from build123d import *

# Parameters (mm, degrees)
SKETCH1_R           = 4
BOSS_EXTRUDE1_DEPTH = 4


with BuildPart() as part:
    # Sketch1 → Boss-Extrude1 (new body)
    with BuildSketch(Plane.XY):
        Polygon((-20, 25), (20, 25), (20, 29), (40, 29), (40, 25), (40, -25), (40, -29), (20, -29), (20, -25), (-20, -25), (-20, -29), (-40, -29), (-40, -25), (-40, 25), (-40, 29), (-20, 29), align=None)
        with Locations((30, 15.5)):
            Circle(SKETCH1_R, mode=Mode.SUBTRACT)
        with Locations(Location((-30, 15.5, 0), (0, 0, 180))):
            Circle(SKETCH1_R, mode=Mode.SUBTRACT)
        with Locations((-30, -15.5)):
            Circle(SKETCH1_R, mode=Mode.SUBTRACT)
        with Locations(Location((30, -15.5, 0), (0, 0, 180))):
            Circle(SKETCH1_R, mode=Mode.SUBTRACT)
    extrude(amount=BOSS_EXTRUDE1_DEPTH)


solid = part.part
Work out the finished part from the listing and answer in its coordinate system (mm). A direction names the side the tool comes from. Round coordinates to 2 decimals unless told otherwise and drop trailing zeros. Order: outer loops, then holes, each group sorted by start corner. A loop starts at its lowest first (then second) coordinate and runs counter-clockwise, first axis right, second up. Notation, with made-up numbers: M -1,-24 L 28,-24 A13 cw 28,-12 Z; hole C 68.25,-5 d4. An arc over 180 degrees is marked long. One line per item, written item: value.
Q1. Determine the mould class of faces 4 (the face through (-40, 0, 2)), 5 (the face through (30, 29, 2)), 6 (the face through (27.05, 18.2, 1.97)) for opening direction X: released by +X, released by -X, zero draft, split by the parting line, or undercut.
Derived:
face 4: released by -X
face 5: zero draft
face 6: undercut
Q2. Straight lines are drawn through the part: line 1 (Y direction, x = 30, z = 2.1); line 2 (X direction, y = 26, z = 0.4); line 3 (Y direction, x = 31, z = 1.55). For each, find the intervals that lie inside material, in ascending order.
Derived:
line 1: -29 to -19.5, -11.5 to 11.5, 19.5 to 29
line 2: -40 to -20, 20 to 40
line 3: -29 to -19.37, -11.63 to 11.63, 19.37 to 29
Q3. Find section C-C on z = 2.9. Write down the section's boundary in (x, y), then the cut area to 3 significant figures.
Derived:
outline: M -40,-29 L -20,-29 L -20,-25 L 20,-25 L 20,-29 L 40,-29 L 40,29 L 20,29 L 20,25 L -20,25 L -20,29 L -40,29 Z; hole C -30,-15.5 d8; hole C -30,15.5 d8; hole C 30,-15.5 d8; hole C 30,15.5 d8
area: 4,120 mm²
Q4. Find section B-B on y = -15.5. Write down the section's boundary in (x, z).
Derived:
outline: M -40,0 L -34,0 L -34,4 L -40,4 Z; M -26,0 L 26,0 L 26,4 L -26,4 Z; M 34,0 L 40,0 L 40,4 L 34,4 Z
Q5. Flat-ended cylindrical pins translate along their axes: pin 1 (2 mm diameter, centred on x = -6.5, z = 3, fed in from +Y); pin 2 (7 mm diameter, centred on x = 30, y = -15.5, fed in from -Z) (3 decimals). Find the tip coordinate at first contact, or state that the pin passes through.
Derived:
pin 1: y = 25
pin 2: through
Q6. For faces 1 (the face through (0, -25, 2)), 2 (the face through (0, 25, 2)), 3 (the face through (40, 0, 2)), determine the directions among +Z, -Z, +X, -X, +Y, -Y from which every point of the face is accessible in a straight line to the end or side of a thin tool.
Derived:
face 1: +Z, -Z, -Y
face 2: +Z, -Z, +Y
face 3: +Z, -Z, +X, +Y, -Y
Q7. Find section A-A on x = 30. Write down the section's boundary in (y, z), then the cut area to 3 significant figures.
Derived:
outline: M -29,0 L -19.5,0 L -19.5,4 L -29,4 Z; M -11.5,0 L 11.5,0 L 11.5,4 L -11.5,4 Z; M 19.5,0 L 29,0 L 29,4 L 19.5,4 Z
area: 168 mm²
Q8. Find section D-D on x = -16. Write down the section's boundary in (y, z), then the cut area to 3 significant figures.
Derived:
outline: M -25,0 L 25,0 L 25,4 L -25,4 Z
area: 200 mm²
